Verification items for the finished model (mm, model axes). Face numbers are marked on the shaded views. Give positions to 0.01 mm unless a question says otherwise; leave off trailing zeros. Order: outer loops, then holes, each group sorted by start corner. A loop starts at its lowest first (then second) coordinate and runs counter-clockwise, first axis right, second up. Notation, with made-up numbers: (68.25, 10) - (119.25, 10) arc R23 cw to (119.25, 29) - close; hole circle Ø10 at (-22, 41.5). An arc over 180 degrees is marked (long way). Answer as a JSON object with one key per item and string values. Group by question number.
(1) Section check B-B (z = 4.65). Record the boundary of the cut face in (x, y).
(2) Section check C-C (y = -5). Record the boundary of the cut face in (x, z).
(3) Section check A-A (x = 30.15). Record the boundary of the cut face in (y, z).
(4) Section check D-D (y = -8.5). Record the boundary of the cut face in (x, z), then the cut area to 3 significant figures.
(5) Thickness scan on line 1 (Y direction, x = 30.15, z = 3.1); line 2 (X direction, y = -2.5, z = 4.1); line 3 (X direction, y = -6.75, z = 1.3). Record the ranges inside material, lowest first.
(6) Mould release check, pull along X, two halves, no side actions. Record for the marked faces 1, 2, 3 and 4: +X half, -X half, draft (parallel to the pull), parting line (faces both ways), or undercut.
```python
from build123d import *

# Parameters (mm, degrees)
F1_DEPTH = 10
F3_R     = 1.25
F4_DEPTH = 5.001


with BuildPart() as f1:
    # F0 (on Front) → F1 (new body)
    with BuildSketch(Plane.XZ):
        with BuildLine():
            Line((4.527255, 5), (0, 5))
            Line((0, 5), (0, 0))
            Line((0, 0), (16.2, 0))
            Line((16.2, 0), (16.2, 5))
            Line((16.2, 5), (13.672745, 5))
            ThreePointArc((13.672745, 5), (9.1, 0.9), (4.527255, 5))
        make_face()
    extrude(amount=F1_DEPTH)

    # F2: F1 across face


with BuildPart() as f1_1:
    add(f1.part)
    add(f1.part.mirror(Plane(origin=(16.2, -5, 2.5), x_dir=(0, 1, 0), z_dir=(1, 0, 0))))

    # F3 (on face) → F4 (cut, through all)
    with BuildSketch(Plane.XY.offset(5)):
        with Locations((2.25, -5)):
            Circle(F3_R)
        with Locations((16.477255, -5)):
            Circle(F3_R)
        with Locations((30.15, -5)):
            Circle(F3_R)
    extrude(amount=-F4_DEPTH, mode=Mode.SUBTRACT)


solid = f1_1.part
```
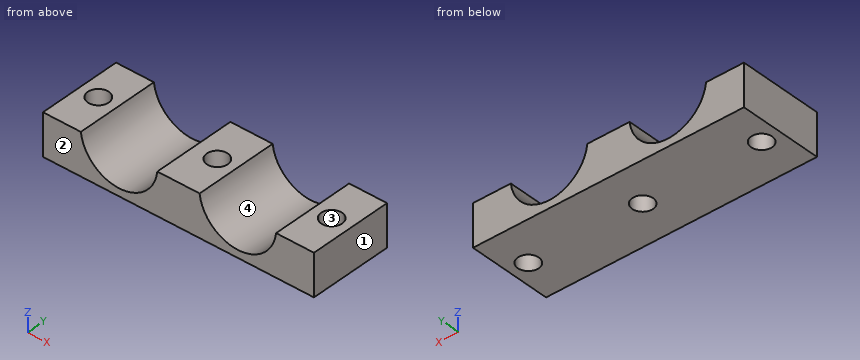
Solutions:
{
 "1": {"outline": "(0, -10) - (4.58, -10) - (4.58, 0) - (0, 0) - close; (13.62, -10) - (18.78, -10) - (18.78, 0) - (13.62, 0) - close; (27.82, -10) - (32.4, -10) - (32.4, 0) - (27.82, 0) - close; hole circle Ø2.5 at (2.25, -5); hole circle Ø2.5 at (16.48, -5); hole circle Ø2.5 at (30.15, -5)"},
 "2": {"outline": "(0, 0) - (1, 0) - (1, 5) - (0, 5) - close; (3.5, 0) - (15.23, 0) - (15.23, 5) - (13.67, 5) arc R4.6 cw to (4.53, 5) - (3.5, 5) - close; (17.73, 0) - (28.9, 0) - (28.9, 5) - (27.87, 5) arc R4.6 cw to (18.73, 5) - (17.73, 5) - close; (31.4, 0) - (32.4, 0) - (32.4, 5) - (31.4, 5) - close"},
 "3": {"outline": "(-10, 0) - (-6.25, 0) - (-6.25, 5) - (-10, 5) - close; (-3.75, 0) - (0, 0) - (0, 5) - (-3.75, 5) - close"},
 "4": {"outline": "(0, 0) - (32.4, 0) - (32.4, 5) - (27.87, 5) arc R4.6 cw to (18.73, 5) - (13.67, 5) arc R4.6 cw to (4.53, 5) - (0, 5) - close", "area": "105 mm2"},
 "5": {"line 1": "y = -10 to -6.25, -3.75 to 0", "line 2": "x = 0 to 4.72, 13.48 to 18.92, 27.68 to 32.4", "line 3": "x = 0 to 7.22, 10.98 to 21.42, 25.18 to 32.4"},
 "6": {"face 1": "+X half", "face 2": "draft", "face 3": "undercut", "face 4": "undercut"}
}
